For this review, take the finished solid that the model builds, in its own axes (mm). A direction names the side the tool comes from. Round coordinates to 2 decimals unless told otherwise and drop trailing zeros. Loops run counter-clockwise (first coordinate to the right, second up) from the corner with the lowest first, then second, coordinate; pieces in that order, holes last.
1. Consider section C-C on z = -59. State the section outline as (x, y) points, then the cut area to 4 significant figures.
2. Consider section A-A on z = 66. State the section outline as (x, y) points, then the cut area to 4 significant figures.
3. Draft analysis for pull direction Z (two halves, no side actions). For faces 5 (the flat face through (2, 58, -87.655)), 6 (the flat face through (2, 55, -115.655)), 7 (the flat face through (2, 65.109, -111)), state which applies: released by +Z, released by -Z, zero draft, split by the parting line, or undercut.
4. Consider section B-B on y = -11. State the section outline as (x, z) points.
5. Clearance check with flat-ended pins moving along their axes: pin 1 Ø5 at (y, z) = (15.11, 131.85) entering from -X; pin 2 Ø1.5 at (x, y) = (3, 39.5) entering from +Z; pin 3 Ø2.5 at (x, z) = (3.5, -114.5) entering from -Y. State where each tip first meets the part, or that it passes through.
6. Tool access review of faces 1 (the flat face through (2, 35, 129.345)), 2 (the flat face through (2, -3, 44.345)), 3 (the flat face through (2, 35, -110.655)), 4 (the cylindrical face through (2.465, -50.687, -67.08)): name each direction out of +Z, -Z, +X, -X, +Y, -Y from which nothing blocks a thin tool from reaching the whole face with its end or side.
7. Consider section D-D on x = 1.25. State how many separate pieces and enclosed holes the cut face has, then the cut area to 3 significant figures.
8. To check wall thickness, follow line 1 along Y through (x, z) = (4.7, 53); line 2 along Z through (x, y) = (3.1, 15); line 3 along Z through (x, y) = (1.2, -16). State the ranges of each line that lie inside material, in increasing order.
from build123d import *

# Parameters (mm, degrees)
SKETCH_1_R      = 4
SKETCH_1_R_2    = 5
SKETCH_1_R_3    = 2.5
SKETCH_1_R_4    = 1.5
EXTRUDE_1_DEPTH = 5


with BuildPart() as part:
    # 草图1 → 凸台-拉伸1 (new body)
    with BuildSketch(Plane(origin=(0, 0, 0), x_dir=(0, 0, -1), z_dir=(1, 0, 0))):
        with BuildLine():
            Line((-84.345470911, -47.190619808), (-84.345470911, -44.190619808))
            ThreePointArc((-84.345470911, -44.190619808), (-83.759684473, -42.776406245), (-82.345470911, -42.190619808))
            Line((-82.345470911, -42.190619808), (63.654529089, -42.190619808))
            ThreePointArc((63.654529089, -42.190619808), (65.068742652, -42.776406245), (65.654529089, -44.190619808))
            Line((65.654529089, -44.190619808), (65.654529089, -47.190619808))
            ThreePointArc((65.654529089, -47.190619808), (67.118995184, -50.726153713), (70.654529089, -52.190619808))
            Line((70.654529089, -52.190619808), (110.654529089, -52.190619808))
            ThreePointArc((110.654529089, -52.190619808), (114.190062995, -50.726153713), (115.654529089, -47.190619808))
            Line((115.654529089, -47.190619808), (115.654529089, -14.890619808))
            Line((115.654529089, -14.890619808), (110.654529089, -14.890619808))
            Line((110.654529089, -14.890619808), (110.654529089, 5.109380192))
            Line((110.654529089, 5.109380192), (115.654529089, 5.109380192))
            Line((115.654529089, 5.109380192), (115.654529089, 25.109380192))
            Line((115.654529089, 25.109380192), (110.654529089, 25.109380192))
            Line((110.654529089, 25.109380192), (110.654529089, 45.109380192))
            Line((110.654529089, 45.109380192), (115.654529089, 45.109380192))
            Line((115.654529089, 45.109380192), (115.654529089, 65.109380192))
            Line((115.654529089, 65.109380192), (105.654529089, 65.109380192))
            ThreePointArc((105.654529089, 65.109380192), (103.533208746, 64.230700536), (102.654529089, 62.109380192))
            Line((102.654529089, 62.109380192), (102.654529089, 53.109380192))
            ThreePointArc((102.654529089, 53.109380192), (101.775849433, 50.988059849), (99.654529089, 50.109380192))
            Line((99.654529089, 50.109380192), (90.654529089, 50.109380192))
            ThreePointArc((90.654529089, 50.109380192), (88.533208746, 50.988059849), (87.654529089, 53.109380192))
            Line((87.654529089, 53.109380192), (87.654529089, 62.109380192))
            ThreePointArc((87.654529089, 62.109380192), (86.775849433, 64.230700536), (84.654529089, 65.109380192))
            Line((84.654529089, 65.109380192), (-103.345470911, 65.109380192))
            ThreePointArc((-103.345470911, 65.109380192), (-105.466791254, 64.230700536), (-106.345470911, 62.109380192))
            Line((-106.345470911, 62.109380192), (-106.345470911, 53.109380192))
            ThreePointArc((-106.345470911, 53.109380192), (-107.224150567, 50.988059849), (-109.345470911, 50.109380192))
            Line((-109.345470911, 50.109380192), (-118.345470911, 50.109380192))
            ThreePointArc((-118.345470911, 50.109380192), (-120.466791254, 50.988059849), (-121.345470911, 53.109380192))
            Line((-121.345470911, 53.109380192), (-121.345470911, 62.109380192))
            ThreePointArc((-121.345470911, 62.109380192), (-122.224150567, 64.230700536), (-124.345470911, 65.109380192))
            Line((-124.345470911, 65.109380192), (-134.345470911, 65.109380192))
            Line((-134.345470911, 65.109380192), (-134.345470911, 45.109380192))
            Line((-134.345470911, 45.109380192), (-129.345470911, 45.109380192))
            Line((-129.345470911, 45.109380192), (-129.345470911, 25.109380192))
            Line((-129.345470911, 25.109380192), (-134.345470911, 25.109380192))
            Line((-134.345470911, 25.109380192), (-134.345470911, 5.109380192))
            Line((-134.345470911, 5.109380192), (-129.345470911, 5.109380192))
            Line((-129.345470911, 5.109380192), (-129.345470911, -14.890619808))
            Line((-129.345470911, -14.890619808), (-134.345470911, -14.890619808))
            Line((-134.345470911, -14.890619808), (-134.345470911, -47.190619808))
            ThreePointArc((-134.345470911, -47.190619808), (-132.881004816, -50.726153713), (-129.345470911, -52.190619808))
            Line((-129.345470911, -52.190619808), (-89.345470911, -52.190619808))
            ThreePointArc((-89.345470911, -52.190619808), (-85.809937005, -50.726153713), (-84.345470911, -47.190619808))
        make_face()
        with Locations((33.654529089, 56.109380192)):
            Circle(SKETCH_1_R, mode=Mode.SUBTRACT)
        with Locations((-52.345470911, 56.109380192)):
            Circle(SKETCH_1_R, mode=Mode.SUBTRACT)
        with Locations((-9.345470911, 43.109380192)):
            Circle(SKETCH_1_R_2, mode=Mode.SUBTRACT)
        with Locations((9.154529089, 43.109380192)):
            Circle(SKETCH_1_R_3, mode=Mode.SUBTRACT)
        with Locations((-27.845470911, 43.109380192)):
            Circle(SKETCH_1_R_3, mode=Mode.SUBTRACT)
        with Locations((113.154529089, 55.109380192)):
            Circle(SKETCH_1_R_4, mode=Mode.SUBTRACT)
        with Locations((-131.845470911, 55.109380192)):
            Circle(SKETCH_1_R_4, mode=Mode.SUBTRACT)
        with Locations((-131.845470911, 15.109380192)):
            Circle(SKETCH_1_R_4, mode=Mode.SUBTRACT)
        with Locations((113.154529089, 15.109380192)):
            Circle(SKETCH_1_R_4, mode=Mode.SUBTRACT)
        with BuildLine():
            Line((-101.345470911, -32.190619808), (-47.345470911, -32.190619808))
            ThreePointArc((-47.345470911, -32.190619808), (-45.224150567, -31.311940151), (-44.345470911, -29.190619808))
            Line((-44.345470911, -29.190619808), (-44.345470911, 24.809380192))
            ThreePointArc((-44.345470911, 24.809380192), (-45.224150567, 26.930700536), (-47.345470911, 27.809380192))
            Line((-47.345470911, 27.809380192), (-101.345470911, 27.809380192))
            ThreePointArc((-101.345470911, 27.809380192), (-103.466791254, 26.930700536), (-104.345470911, 24.809380192))
            Line((-104.345470911, 24.809380192), (-104.345470911, -29.190619808))
            ThreePointArc((-104.345470911, -29.190619808), (-103.466791254, -31.311940151), (-101.345470911, -32.190619808))
        make_face(mode=Mode.SUBTRACT)
    extrude(amount=EXTRUDE_1_DEPTH)


solid = part.part
Resolved:
1. outline: (0, -42.19) - (5, -42.19) - (5, 65.11) - (0, 65.11) - close
1. area: 536.5 mm2
2. outline: (0, -42.19) - (5, -42.19) - (5, -32.19) - (0, -32.19) - close; (0, 27.81) - (5, 27.81) - (5, 65.11) - (0, 65.11) - close
2. area: 236.5 mm2
3. face 5: undercut
3. face 6: released by -Z
3. face 7: zero draft
4. outline: (0, -110.65) - (5, -110.65) - (5, 44.35) - (0, 44.35) - close; (0, 104.35) - (5, 104.35) - (5, 129.35) - (0, 129.35) - close
5. pin 1: stops at x = 0
5. pin 2: stops at z = 129.35
5. pin 3: stops at y = -51.46
6. face 1: +Z, +X, -X
6. face 2: +X, -X
6. face 3: -Z, +X, -X
6. face 4: +X, -X, -Y
7. separate pieces: 1
7. enclosed holes: 10
7. area: 23,100 mm2
8. line 1: y = -42.19 to -32.19, 27.81 to 52.16, 60.06 to 65.11
8. line 2: z = -115.65 to -114.65, -111.66 to 44.35, 104.35 to 130.35, 133.34 to 134.35
8. line 3: z = -115.65 to 44.35, 104.35 to 134.35
